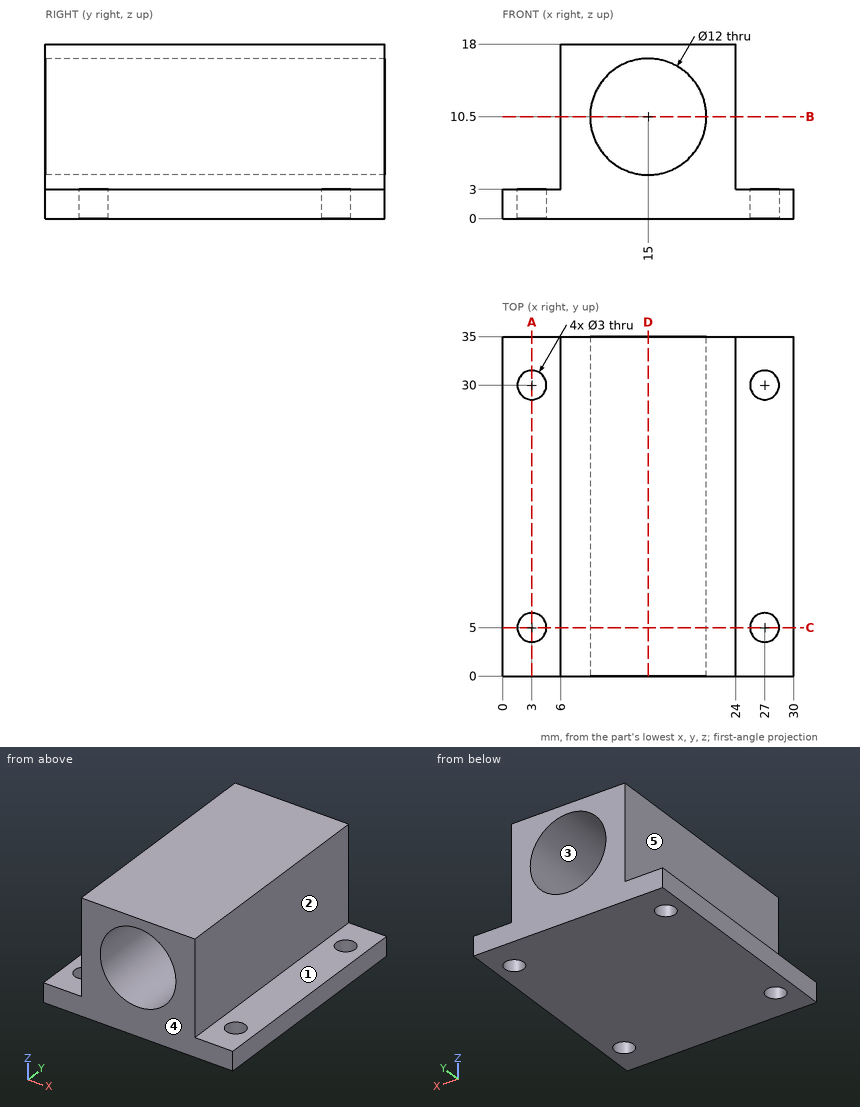
Job drawing, mm, ordinate dimensions from the low corner. One solid piece. A direction names the side the tool comes from. Give positions to 0.01 mm unless a question says otherwise; leave off trailing zeros. Write each loop counter-clockwise with the first axis right and the second up, starting at its lowest first coordinate (ties: lowest second). Pieces come first, ordered by that corner, then holes. Notation, with made-up numbers: (25.5, 28) - (71.5, 28) arc R26 cw to (71.5, 67) - close; hole circle Ø1 at (-3, 0). An arc over 180 degrees is marked (long way). Use one line per item in the form item = value. Start each with the question number.
1. Probe line 1 (Y direction, x = 27, z = 1.35); line 2 (Z direction, x = 15, y = 19); line 3 (X direction, y = 6, z = 1.5). List the from-to ranges inside material, lowest first. Write a range as [from, to].
2. Band-saw the part on C-C on y = 5. Write the cut outline in (x, z), plus the area to 3 significant figures.
3. 3-axis set-ups, long thin cutter, end or side, ignore diameter. For the marked faces 4 and 5: which of +Z, -Z, +X, -X, +Y, -Y reach the whole face in a straight line?
4. Band-saw the part on A-A on x = 3. Write the cut outline in (y, z).
5. Band-saw the part on D-D on x = 15. Write the cut outline in (y, z).
6. Band-saw the part on B-B on z = 10.5. Write the cut outline in (x, y).
7. Two-plate mould, pull along Z, no slides. Class the marked faces 1, 2 and 3: released by +Z, released by -Z, zero draft, split by the parting line, or undercut.
8. Drop flat-ended pins along their axis: pin 1 Ø2.5 at (x, y) = (27, 5) entering from +Z; pin 2 Ø3 at (x, y) = (4, 13) entering from +Z; pin 3 Ø1 at (y, z) = (26, 5.5) entering from +X; pin 4 Ø7.5 at (y, z) = (11.5, 13.5) entering from -X. Give the stop position or say it passes through.
Conclusion:
q1.line_1 = [0, 3.5], [6.5, 28.5], [31.5, 35]
q1.line_2 = [0, 4.5], [16.5, 18]
q1.line_3 = [0, 1.88], [4.12, 25.88], [28.12, 30]
q2.outline = (0, 0) - (1.5, 0) - (1.5, 3) - (0, 3) - close; (4.5, 0) - (25.5, 0) - (25.5, 3) - (24, 3) - (24, 18) - (6, 18) - (6, 3) - (4.5, 3) - close; (28.5, 0) - (30, 0) - (30, 3) - (28.5, 3) - close; hole circle Ø12 at (15, 10.5)
q2.area = 229 mm²
q3.face_4 = +Z, -Z, +X, -X, -Y
q3.face_5 = +Z, -X, +Y, -Y
q4.outline = (0, 0) - (3.5, 0) - (3.5, 3) - (0, 3) - close; (6.5, 0) - (28.5, 0) - (28.5, 3) - (6.5, 3) - close; (31.5, 0) - (35, 0) - (35, 3) - (31.5, 3) - close
q5.outline = (0, 0) - (35, 0) - (35, 4.5) - (0, 4.5) - close; (0, 16.5) - (35, 16.5) - (35, 18) - (0, 18) - close
q6.outline = (6, 0) - (9, 0) - (9, 35) - (6, 35) - close; (21, 0) - (24, 0) - (24, 35) - (21, 35) - close
q7.face_1 = released by +Z
q7.face_2 = zero draft
q7.face_3 = undercut
q8.pin_1 = through
q8.pin_2 = 3
q8.pin_3 = 24
q8.pin_4 = 6
